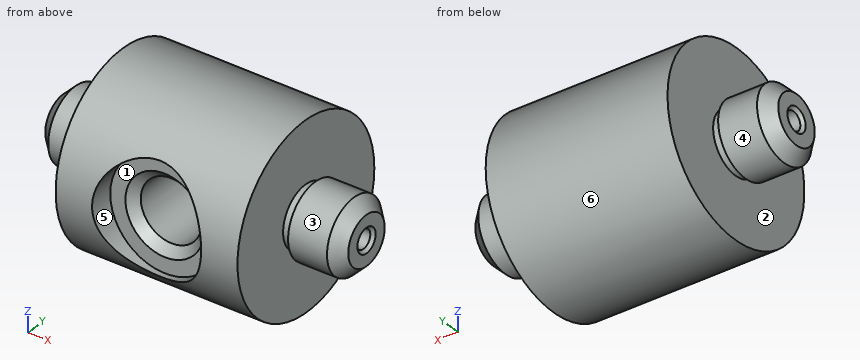
Autodesk Inventor part; units mm, degrees
ref_plane "YZ Plane" through (0, 0, 0) normal (1, 0, 0) x (0, 1, 0)
ref_plane "XZ Plane" through (0, 0, 0) normal (0, 1, 0) x (-1, 0, 0)
ref_plane "XY Plane" through (0, 0, 0) normal (0, 0, 1) x (1, 0, 0)
sketch "Sketch1" plane through (0, 0, 0) normal (0, 0, 1) x (1, 0, 0)
  line L0 (-35, 0) -> (35, 0) construction
  line L1 (0, -21) -> (0, 21) construction
  line L2 (0, 15) -> (-15, 15)
  line L3 (-15, 15) -> (-15, 5)
  line L4 (-15, 5) -> (-16, 5)
  line L5 (-16, 5) -> (-16.5774, 6)
  line L6 (-16.5774, 6) -> (-25, 6)
  line L7 (-25, 6) -> (-25, 0)
  line L8 (0, 15) -> (15, 15)
  line L9 (15, 15) -> (15, 5)
  line L10 (15, 5) -> (16, 5)
  line L11 (16, 5) -> (16.5774, 6)
  line L12 (16.5774, 6) -> (25, 6)
  line L13 (25, 6) -> (25, 0)
  line L14 (0, -15) -> (-15, -15)
  line L15 (-15, -15) -> (-15, -5)
  line L16 (-15, -5) -> (-16, -5)
  line L17 (-16, -5) -> (-16.5774, -6)
  line L18 (-16.5774, -6) -> (-25, -6)
  line L19 (-25, -6) -> (-25, 0)
  line L20 (15, -15) -> (15, -5)
  line L21 (15, -5) -> (16, -5)
  line L22 (16, -5) -> (16.5774, -6)
  line L23 (16.5774, -6) -> (25, -6)
  line L24 (25, -6) -> (25, 0)
  line L25 (0, -15) -> (15, -15)
  line L26 (-9, -15) -> (-9, -11)
  line L27 (-9, -11) -> (-5, -11)
  line L28 (-5, -11) -> (-5, 8)
  line L29 (-5, 8) -> (0, 11.0043)
  line L30 (0, 11.0043) -> (0, -15)
  line L31 (-25, 0) -> (25, 0)
  line L32 (-25, 1.5) -> (25, 1.5)
  point P0 (0, 0)
  dimension "d0" = 30
  dimension "d1" = 12
  dimension "d3" = 8.4227
  dimension "d5" = 60
  dimension "d6" = 10
  dimension "d7" = 30
  dimension "d8" = 50
  dimension "d9" = 59
  dimension "d10" = 10
  dimension "d11" = 4
  dimension "d12" = 18
  dimension "d13" = 23
  dimension "d23" = 3
  dimension "d27" = 10
  dimension "d29" = 1
revolve "Revolution1" add sketch "Sketch1" angle 360 about axis through (-25, 0, 0) along (1, 0, 0) contours L8 L9 L10 L11 L12 L13 L32 L30 L29 L28 L7 L6 L5 L4 L3 L2 | L28 L29 L30 L32
revolve "Revolution2" cut sketch "Sketch1" angle 360 about axis through (0, 11.0043, 0) along (0, -1, 0) contours L32 L30 L31 L28 | L28 L29 L30 L32 | L31 L30 L14 L26 L27 L28
thread "Thread2"
chamfer "Chamfer1" distance 2 angle 45 2 edges at (-25, -6, 0) (25, -6, 0)
chamfer "Chamfer2" distance 0.5 angle 45 2 edges at (-25, -1.5, 0) (25, -1.5, 0)
sketch "Sketch2" plane through (0, -11, 0) normal (0, -1, 0) x (0, 0, -1)
  circle A0 centre (0, 0) radius 5
  point P0 (0, 0)
hole "Hole1" at (0, -11, 0) direction (0, 1, 0) diameter 10.106 depth 20 tip angle 118 countersink diameter 13 countersink angle 90
properties part number "HM1-002" material "Steel, Alloy"
Geometry check sheet. Reference: the model listing, model coordinates, mm. Face numbers are marked on the shaded views. A direction names the side the tool comes from. Give positions to 0.01 mm unless a question says otherwise; leave off trailing zeros. Order: outer loops, then holes, each group sorted by start corner. A loop starts at its lowest first (then second) coordinate and runs counter-clockwise, first axis right, second up. Notation, with made-up numbers: (52, 71.25) - (84, 71.25) arc R13 cw to (84, 85.25) - close; hole circle Ø3 at (-24, -7.5). An arc over 180 degrees is marked (long way). Use one line per item in the form item = value.
1) Sectioned sample at A-A (x = -19). Record the boundary of the cut face in (y, z).
Working result:
outline = circle Ø12 at (0, 0); hole circle Ø3 at (0, 0)
2) Sectioned sample at B-B (z = -7.5). Record the boundary of the cut face in (x, y).
Working result:
outline = (-15, -12.99) - (-4.97, -12.99) - (-4.97, -11) - (4.97, -11) - (4.97, -12.99) - (15, -12.99) - (15, 12.99) - (-15, 12.99) - close
3) Sectioned sample at D-D (z = 8). Record the boundary of the cut face in (x, y), and give its area (3 significant figures).
Working result:
outline = (-15, -12.69) - (-4.12, -12.69) - (-4.12, -11) - (4.12, -11) - (4.12, -12.69) - (15, -12.69) - (15, 12.69) - (-15, 12.69) - close
area = 747 mm^2
4) Depth check by flat-ended pin: pin 1 Ø1.5 at (y, z) = (9, 11.5) entering from +X; pin 2 Ø2 at (y, z) = (-8.5, 4) entering from -X; pin 3 Ø10 at (x, z) = (19, 5) entering from -Y. Enter the tip coordinate at first touch or a pass-through.
Working result:
pin_1 = 15
pin_2 = -15
pin_3 = -14.87
5) Access from +Z, -Z, +X, -X, +Y, -Y to the whole of each face (thin tool, end or side, straight path). Record for the marked faces 4, 5 and 6.
Working result:
face_4 = -X
face_5 = -Y
face_6 = +X, -X
6) Material ranges on probe 1 along X at (y, z) = (4.5, -3); probe 2 along X at (y, z) = (5, -1.5); probe 3 along X at (y, z) = (5, -10), recorded low to high. Write a range as from..to.
Working result:
probe_1 = -23.59..-16.24, -15..-4.07, 4.07..15, 16.24..23.59
probe_2 = -23.78..-16.13, -15..-4.83, 4.83..15, 16.13..23.78
probe_3 = -15..15
7) Sectioned sample at C-C (x = -10). Record the boundary of the cut face in (y, z).
Working result:
outline = circle Ø30 at (0, 0); hole circle Ø3 at (0, 0)
8) Draft check along Z on the marked faces 1, 2 and 3. Enter one of: released by +Z, released by -Z, zero draft, split by the parting line, or undercut.
Working result:
face_1 = undercut
face_2 = zero draft
face_3 = split by the parting line
